```python
from build123d import *

# Parameters (mm, degrees)
BOSS_EXTRUDE1_DEPTH = 12.7
CUT_EXTRUDE2_DEPTH  = 15.24
CHAMFER1_SIZE       = 2.54


with BuildPart() as part:
    # Sketch1 → Boss-Extrude1 (new body)
    with BuildSketch(Plane(origin=(0, 0, 0), x_dir=(1, 0, 0), z_dir=(0, 1, 0))):
        with BuildLine():
            Line((65.393705137, 0), (95.25, 0))
            ThreePointArc((95.25, 0), (92.004434954, -24.652514046), (82.48891971, -47.625))
            Line((82.48891971, -47.625), (56.632609896, -32.696852568))
            ThreePointArc((56.632609896, -32.696852568), (59.12802761, -27.932293541), (61.223461988, -22.978780943))
            Line((61.223461988, -22.978780943), (5.214104757, -7.971118904))
            ThreePointArc((5.214104757, -7.971118904), (1.505608988, -9.405252074), (-2.465251405, -9.200443495))
            Line((-2.465251405, -9.200443495), (-10.84710618, -40.48195138))
            Line((-10.84710618, -40.48195138), (-52.758242936, -29.251896132))
            ThreePointArc((-52.758242936, -29.251896132), (-58.269475471, 15.613258896), (-31.064030575, 51.712006627))
            Line((-31.064030575, 51.712006627), (10.84710618, 40.48195138))
            Line((10.84710618, 40.48195138), (2.465251405, 9.200443495))
            ThreePointArc((2.465251405, 9.200443495), (6.006521669, 7.392382731), (8.501106629, 4.296139089))
            Line((8.501106629, 4.296139089), (64.510463861, -10.711522949))
            ThreePointArc((64.510463861, -10.711522949), (65.172520756, -5.373938012), (65.393705137, 0))
        make_face()
    extrude(amount=BOSS_EXTRUDE1_DEPTH)

    # Sketch2 → Revolve1 (revolve)
    with BuildSketch(Plane.XY, mode=Mode.PRIVATE) as revolve1_sk:
        with BuildLine():
            Line((6.985, 0), (0, 0))
            Line((0, 0), (0, -12.192))
            Line((0, -12.192), (1.905, -12.192))
            ThreePointArc((1.905, -12.192), (5.497102448, -10.704102448), (6.985, -7.112))
            Line((6.985, -7.112), (6.985, 0))
        make_face()
    revolve(revolve1_sk.sketch.rotate(Axis((0, -12.192, 0), (0, 1, 0)), 90), axis=Axis((0, -12.192, 0), (0, 1, 0)))

    # Sketch5 → Cut-Extrude2 (cut)
    with BuildSketch(Plane(origin=(0, 12.7, 0), x_dir=(1, 0, 0), z_dir=(0, 1, 0))):
        Polygon((3.007156908, 3.007156908), (-1.100695821, 4.107852729), (-4.107852729, 1.100695821), (-3.007156908, -3.007156908), (1.100695821, -4.107852729), (4.107852729, -1.100695821), align=None)
    extrude(amount=-CUT_EXTRUDE2_DEPTH, mode=Mode.SUBTRACT)

    # Chamfer1
    chamfer1_edges = [part.edges().sort_by_distance(p)[0] for p in [
        (80.321852568, 0, 0),
        (80.321852568, 12.7, 0),
    ]]
    chamfer(chamfer1_edges, length=CHAMFER1_SIZE)


solid = part.part
```
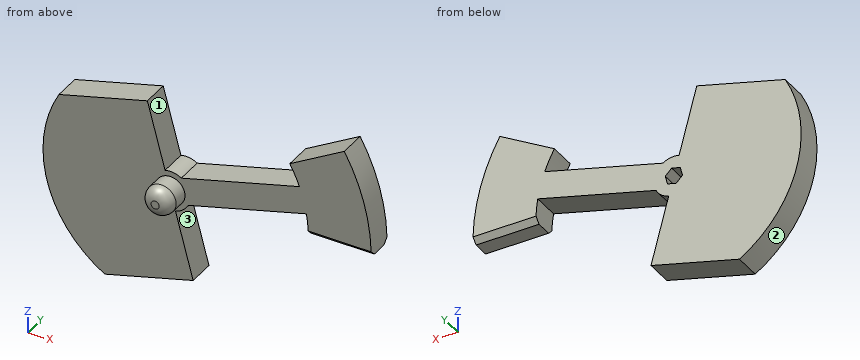
Build history of the part. All positions in model axes, mm. Face numbers are marked on the shaded views. Give positions to 0.01 mm unless a question says otherwise; leave off trailing zeros. Loops run counter-clockwise (first coordinate to the right, second up) from the corner with the lowest first, then second, coordinate; pieces in that order, holes last.
Item 1: Flat gauge pins, fed straight in: pin 1 (4 mm diameter, centred on x = 1, z = 0.5, fed in from +Y); pin 2 (8.5 mm diameter, centred on x = 81.5, y = 6, fed in from -Z); pin 3 (3 mm diameter, centred on x = 7.5, y = 6.5, fed in from -Z); pin 4 (10 mm diameter, centred on x = 6, z = 15.5, fed in from +Y). Where does each tip first touch, or does it go through?
Answers follow:
pin 1: stops at y = -2.54
pin 2: stops at z = 0
pin 3: stops at z = -41.78
pin 4: passes through
Item 2: Drill centre lines: line 1 (Y direction, x = 21, z = 9); line 2 (X direction, y = 11, z = -36); line 3 (X direction, y = 0.5, z = -8.5). Where is each one in solid material? Low to high.
Answers follow:
line 1: y = 0 to 12.7
line 2: x = -48.41 to 9.65
line 3: x = -59.72 to 4.3
Item 3: Slice it at B-B, the plane y = 4.5. List the corners of the cut face in (x, z) (3 decimals), and give its area (3 significant figures).
Answers follow:
outline: (-52.758, 29.252) arc R60.325 ccw to (-31.064, -51.712) - (10.847, -40.482) - (2.465, -9.2) arc R9.525 ccw to (8.501, -4.296) - (64.51, 10.712) arc R65.394 cw to (65.394, 0) - (95.25, 0) arc R95.25 ccw to (82.489, 47.625) - (56.633, 32.697) arc R65.394 cw to (61.223, 22.979) - (5.214, 7.971) arc R9.525 ccw to (-2.465, 9.2) - (-10.847, 40.482) - close; hole (-4.108, -1.101) - (-1.101, -4.108) - (3.007, -3.007) - (4.108, 1.101) - (1.101, 4.108) - (-3.007, 3.007) - close
area: 6,680 mm2
Item 4: Pull direction X, two halves, no side cores. Call the marked faces 1, 2 and 3: released by +X, released by -X, zero draft, split by the parting line, or undercut.
Answers follow:
face 1: undercut
face 2: released by -X
face 3: released by +X
Item 5: Slice it at A-A, the plane z = 20. List the corners of the cut face in (x, y), and give its area (3 significant figures).
Answers follow:
outline: (-56.91, 0) - (-5.36, 0) - (-5.36, 12.7) - (-56.91, 12.7) - close; (50.11, 0) - (93.13, 0) - (93.13, 12.7) - (50.11, 12.7) - close
area: 1,200 mm2
Item 6: Slice it at D-D, the plane z = -45. List the corners of the cut face in (x, y), and give its area (3 significant figures).
Answers follow:
outline: (-40.18, 0) - (-6.01, 0) - (-6.01, 12.7) - (-40.18, 12.7) - close
area: 434 mm2
Item 7: Slice it at C-C, the plane x = -14.5. List the corners of the cut face in (y, z).
Answers follow:
outline: (0, -47.27) - (12.7, -47.27) - (12.7, 39.5) - (0, 39.5) - close
